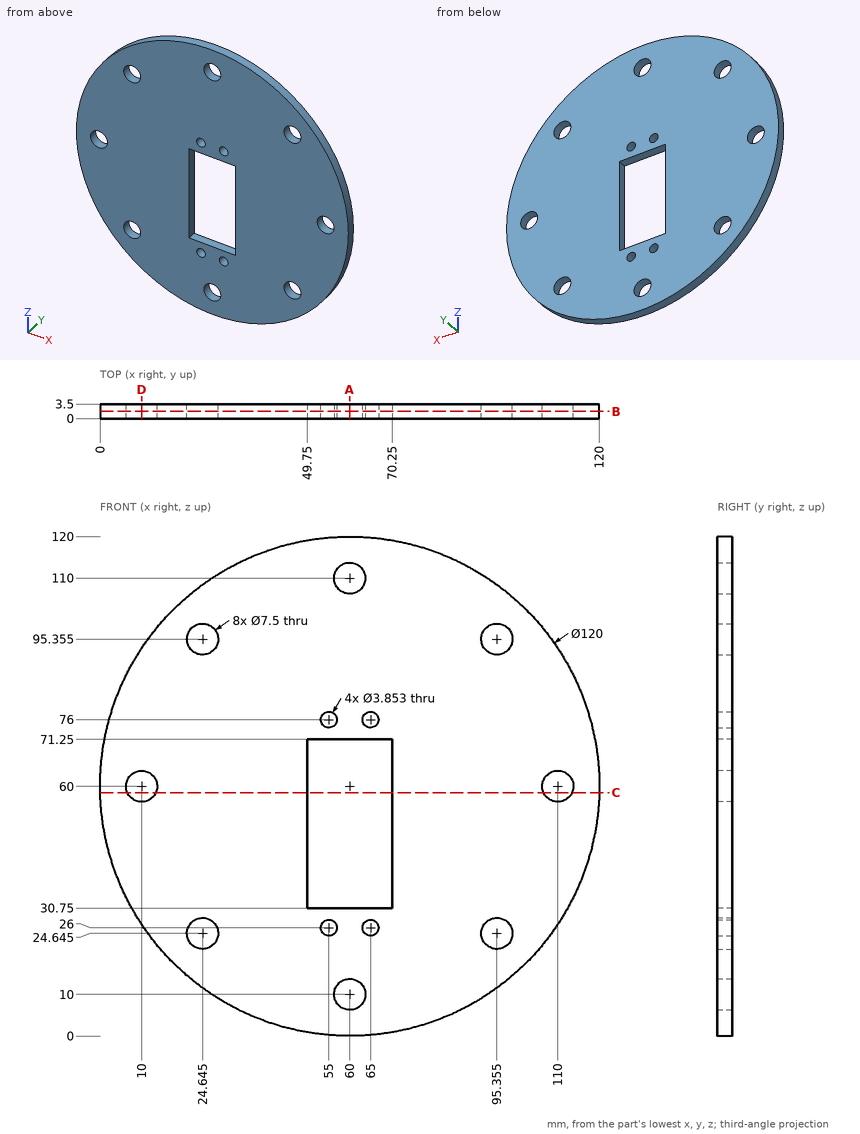
Source: three-view drawing plus pictorial views. Frame: mm from the lowest corner of the part. Coordinates: 2 decimals unless noted, no trailing zeros. Loops run counter-clockwise (first coordinate to the right, second up) from the corner with the lowest first, then second, coordinate; pieces in that order, holes last. Notation, with made-up numbers: (5, 38) - (18, 38) arc R28 cw to (18, 71) - close; hole circle Ø9 at (-32.75, 34.5). An arc over 180 degrees is marked (long way). One line per question, with ' | ' between items.
1) Section D-D, the plane x = 10. Return loops of the section in (y, z).
Report:
outline: (0, 26.83) - (3.5, 26.83) - (3.5, 56.25) - (0, 56.25) - close; (0, 63.75) - (3.5, 63.75) - (3.5, 93.17) - (0, 93.17) - close
2) Line query: line 1 along X through (y, z) = (2.15, 60); line 2 along Z through (x, y) = (60, 2.25); line 3 along Z through (x, y) = (27.5, 2.15) (1 decimal). Output: solid intervals per line, ascending.
Report:
line 1: x = 0 to 6.25, 13.75 to 49.75, 70.25 to 106.25, 113.75 to 120 | line 2: z = 0 to 6.25, 13.75 to 30.75, 71.25 to 106.25, 113.75 to 120 | line 3: z = 9.6 to 22.2, 27.1 to 92.9, 97.8 to 110.4
3) First-contact query: P1, Ø1, axis at y = 2, z = 12.5, coming from the +X side (1 decimal); P2, Ø1.8, axis at x = 55.5, y = 2, coming from the +Z side; P3, Ø1.8, axis at y = 1.5, z = 45.5, coming from the -X side. Flat tips, straight axial feed; report the tip coordinate or a pass-through.
Report:
P1: stops at x = 97.3 | P2: stops at z = 119.89 | P3: stops at x = 1.56
4) Section A-A, the plane x = 60. Return loops of the section in (y, z), then the cut area to 3 significant figures.
Report:
outline: (0, 0) - (3.5, 0) - (3.5, 6.25) - (0, 6.25) - close; (0, 13.75) - (3.5, 13.75) - (3.5, 30.75) - (0, 30.75) - close; (0, 71.25) - (3.5, 71.25) - (3.5, 106.25) - (0, 106.25) - close; (0, 113.75) - (3.5, 113.75) - (3.5, 120) - (0, 120) - close | area: 226 mm²
5) Section C-C, the plane z = 58.5. Return loops of the section in (x, y), then the cut area to 3 significant figures.
Report:
outline: (0.02, 0) - (6.56, 0) - (6.56, 3.5) - (0.02, 3.5) - close; (13.44, 0) - (49.75, 0) - (49.75, 3.5) - (13.44, 3.5) - close; (70.25, 0) - (106.56, 0) - (106.56, 3.5) - (70.25, 3.5) - close; (113.44, 0) - (119.98, 0) - (119.98, 3.5) - (113.44, 3.5) - close | area: 300 mm²
6) Section B-B, the plane y = 1.7. Give the number of separate pieces and of enclosed holes in the cut face, then the cut area to 3 significant figures.
Report:
separate pieces: 1 | enclosed holes: 13 | area: 10,100 mm²
